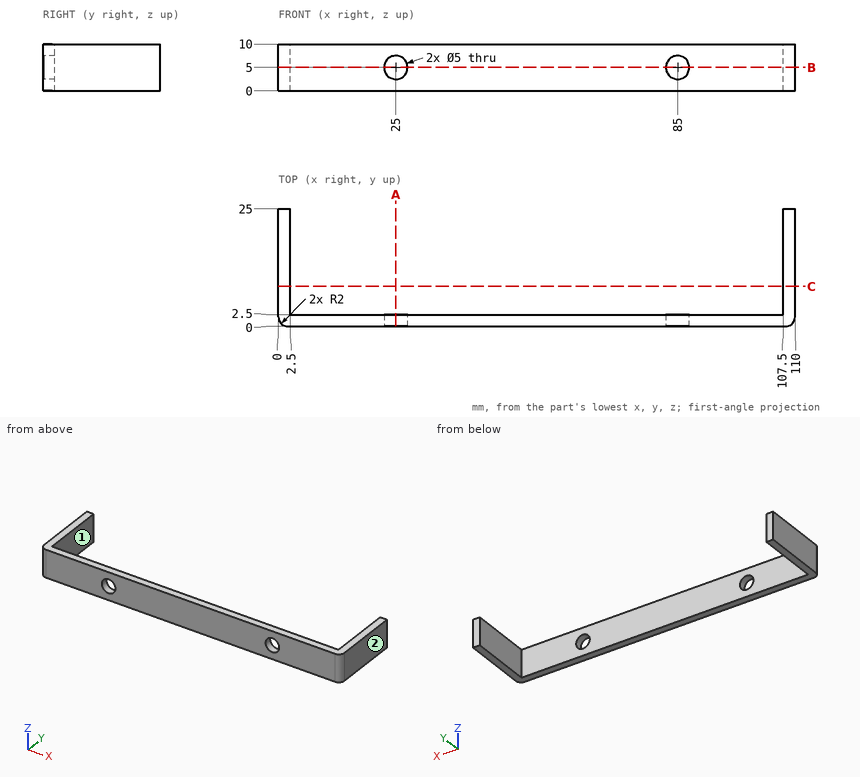
Geometry check sheet. Reference: drawing and pictorial views, mm from the part's lowest x, y, z. A direction names the side the tool comes from. Give positions to 0.01 mm unless a question says otherwise; leave off trailing zeros. Write each loop counter-clockwise with the first axis right and the second up, starting at its lowest first coordinate (ties: lowest second). Pieces come first, ordered by that corner, then holes. Notation, with made-up numbers: (54.25, -28) - (99.25, -28) arc R16 ccw to (99.25, -5) - close; hole circle Ø2 at (32, 36.25). An arc over 180 degrees is marked (long way). Put each result on its own line as item: value.
Q1. Scan lines: probe 1 along X at (y, z) = (23.25, 4.25); probe 2 along Y at (x, z) = (61.5, 1.5); probe 3 along Z at (x, y) = (85, 0.7). Record each from-to range of solid material in increasing order. Write a range as from..to.
Result:
probe 1: 0..2.5, 107.5..110
probe 2: 0..2.5
probe 3: 0..2.5, 7.5..10
Q2. Section check B-B on z = 5. Record the cut outline in (x, y), and give its area (3 significant figures).
Result:
outline: (0, 2) arc R2 ccw to (2, 0) - (22.5, 0) - (22.5, 2.5) - (2.5, 2.5) - (2.5, 25) - (0, 25) - close; (27.5, 0) - (82.5, 0) - (82.5, 2.5) - (27.5, 2.5) - close; (87.5, 0) - (108, 0) arc R2 ccw to (110, 2) - (110, 25) - (107.5, 25) - (107.5, 2.5) - (87.5, 2.5) - close
area: 361 mm2
Q3. Set-up check for the marked faces 1 and 2: record each of +Z, -Z, +X, -X, +Y, -Y from which the full face is reachable in a straight line by a thin tool's end or side.
Result:
face 1: +Z, -Z, +Y
face 2: +Z, -Z, +X, +Y, -Y
Q4. Section check A-A on x = 25. Record the cut outline in (y, z), and give its area (3 significant figures).
Result:
outline: (0, 0) - (2.5, 0) - (2.5, 2.5) - (0, 2.5) - close; (0, 7.5) - (2.5, 7.5) - (2.5, 10) - (0, 10) - close
area: 12.5 mm2
Q5. Depth check by flat-ended pin: P1, Ø6, axis at x = 25, z = 5, coming from the +Y side; P2, Ø10, axis at x = 42.5, y = 12, coming from the +Z side (3 decimals); P3, Ø5, axis at y = 8, z = 6.5, coming from the -X side. Enter the tip coordinate at first touch or a pass-through.
Result:
P1: y = 2.5
P2: through
P3: x = 0
Q6. Section check C-C on y = 8.5. Record the cut outline in (x, z).
Result:
outline: (0, 0) - (2.5, 0) - (2.5, 10) - (0, 10) - close; (107.5, 0) - (110, 0) - (110, 10) - (107.5, 10) - close
